from build123d import *

# Parameters (mm, degrees)
F1_R     = 12.7
F2_DEPTH = 25.4
F0_R     = 59.055
F3_DEPTH = 6.35
F4_R     = 3.683
F5_DEPTH = 6.351
F6_R     = 59.055
F6_R_2   = 54.61
F7_DEPTH = 1.27


with BuildPart() as f2:
    # F1 (on Front) → F2 (new body)
    with BuildSketch(Plane.XZ):
        Circle(F1_R)
    extrude(amount=F2_DEPTH)

    # F0 (on Front) → F3 (join)
    with BuildSketch(Plane.XZ):
        Circle(F0_R)
    extrude(amount=-F3_DEPTH)

    # F4 (on Front) → F5 (cut, through all)
    with BuildSketch(Plane.XZ):
        with Locations((17.78, -5.192251)):
            Circle(F4_R)
    extrude(amount=-F5_DEPTH, mode=Mode.SUBTRACT)

    # F6 (on face) → F7 (join)
    with BuildSketch(Plane(origin=(0, 6.35, 0), x_dir=(-1, 0, 0), z_dir=(0, 1, 0))):
        Circle(F6_R)
        Circle(F6_R_2, mode=Mode.SUBTRACT)
    extrude(amount=F7_DEPTH)


solid = f2.part
Could you check a few things on this model? Use its own coordinates, in mm. A direction names the side the tool comes from. Round coordinates to 2 decimals unless told otherwise and drop trailing zeros. Order: outer loops, then holes, each group sorted by start corner. A loop starts at its lowest first (then second) coordinate and runs counter-clockwise, first axis right, second up.
Q1. Please list where these lines run through material, in increasing order: probe 1 along Z at (x, y) = (0, 7.1) (3 decimals); probe 2 along Z at (x, y) = (0, 6) (3 decimals); probe 3 along Y at (x, z) = (-22, 11.5).
Geometry says:
probe 1: z = -59.055 to -54.61, 54.61 to 59.055
probe 2: z = -59.055 to 59.055
probe 3: y = 0 to 6.35
Q2. Imagine slicing it at D-D, the plane y = -17.5. List the corners of the cut face in (x, z) for me, then the cut area to 3 significant figures.
Geometry says:
outline: circle Ø25.4 at (0, 0)
area: 507 mm2
Q3. Thinking about a two-plate mould opening in X: for faces 1 (the face through (-1, 6.35, 1)), 2 (the face through (-2.75, -12.52, -12.4)), 3 (the face through (15.07, 3.13, -2.7)), 4 (the face through (-1, 0, 14)), which applies, released by +X, released by -X, zero draft, split by the parting line, or undercut?
Geometry says:
face 1: undercut
face 2: split by the parting line
face 3: undercut
face 4: zero draft
Q4. Imagine slicing it at B-B, the plane z = 0. List the corners of the cut face in (x, y) for me (3 decimals).
Geometry says:
outline: (-59.055, 0) - (-12.7, 0) - (-12.7, -25.4) - (12.7, -25.4) - (12.7, 0) - (59.055, 0) - (59.055, 7.62) - (54.61, 7.62) - (54.61, 6.35) - (-54.61, 6.35) - (-54.61, 7.62) - (-59.055, 7.62) - close
Q5. Imagine slicing it at A-A, the plane x = 17.78. List the corners of the cut face in (y, z) for me.
Geometry says:
outline: (0, -56.31) - (7.62, -56.31) - (7.62, -51.63) - (6.35, -51.63) - (6.35, -8.88) - (0, -8.88) - close; (0, -1.51) - (6.35, -1.51) - (6.35, 51.63) - (7.62, 51.63) - (7.62, 56.31) - (0, 56.31) - close
Q6. Which directions (+Z, -Z, +X, -X, +Y, -Y) give clear straight access to the entire face, cutting with the end or side of a thin tool? Please do faces 5 (the face through (7.109, 6.976, 54.145)), 6 (the face through (0, -25.4, 0)).
Geometry says:
face 5: +Y
face 6: +Z, -Z, +X, -X, -Y
Q7. Imagine slicing it at C-C, the plane x = 0. List the corners of the cut face in (y, z) for me (3 decimals), then the cut area to 3 significant figures.
Geometry says:
outline: (-25.4, -12.7) - (0, -12.7) - (0, -59.055) - (7.62, -59.055) - (7.62, -54.61) - (6.35, -54.61) - (6.35, 54.61) - (7.62, 54.61) - (7.62, 59.055) - (0, 59.055) - (0, 12.7) - (-25.4, 12.7) - close
area: 1,410 mm2
Q8. I'm going to push flat-ended pins straight in: P1, Ø8, axis at x = 20.5, y = -8, coming from the -Z side; P2, Ø6, axis at x = -32.5, z = 24, coming from the +Y side; P3, Ø6, axis at x = 35.5, z = 16.5, coming from the -Y side; P4, Ø10, axis at y = -8.5, z = 5.5, coming from the -X side. Where does each tip first touch, or does it pass through?
Geometry says:
P1: passes through
P2: stops at y = 6.35
P3: stops at y = 0
P4: stops at x = -12.69
